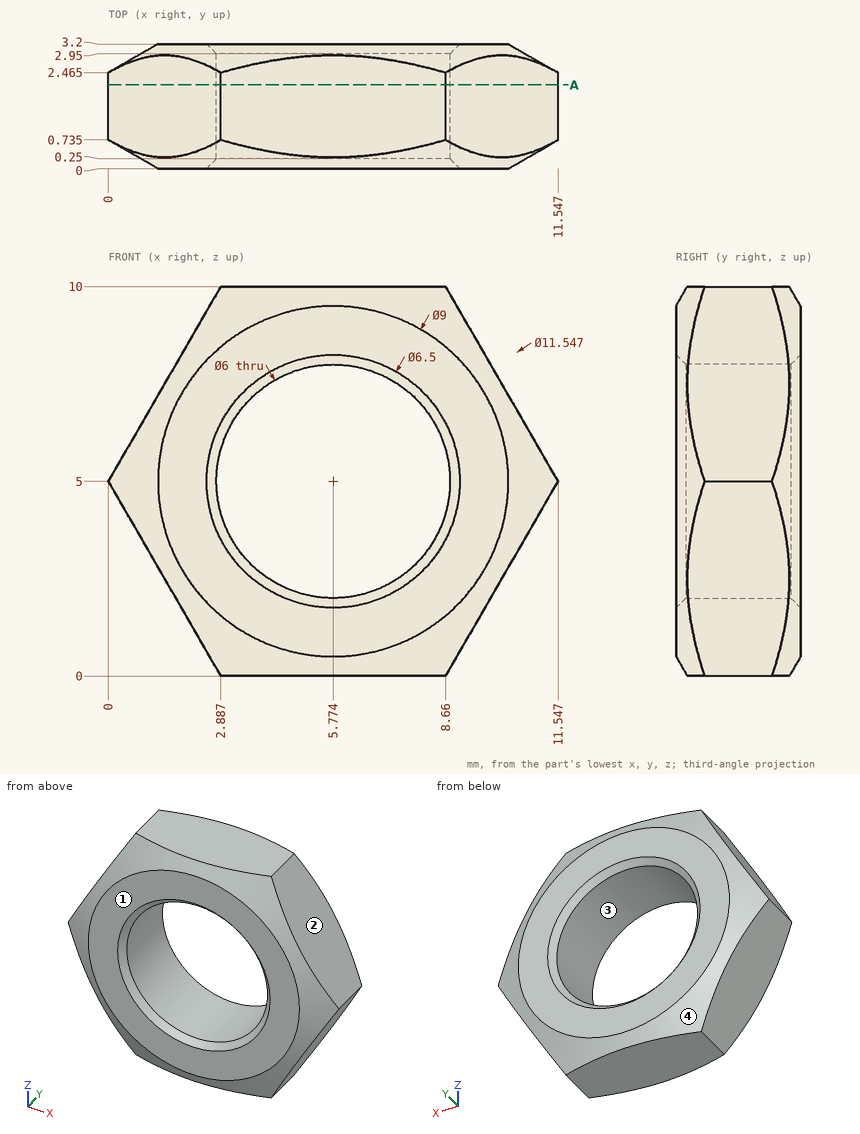
Can you work these out from the drawing? Everything is in mm from the part's minimum corner. Coordinates: 2 decimals unless noted, no trailing zeros. Loops run counter-clockwise (first coordinate to the right, second up) from the corner with the lowest first, then second, coordinate; pieces in that order, holes last. Notation, with made-up numbers: (20, 26.5) - (70, 26.5) arc R30 cw to (70, 56.5) - close; hole circle Ø11 at (-4, -9.5). An arc over 180 degrees is marked (long way). Use a Markdown table: item, result.
Item 1: If I drill on probe 1 along Z at (x, y) = (5.75, 1.1); probe 2 along Z at (x, y) = (4, 2.2); probe 3 along X at (y, z) = (1.55, 4.5) (1 decimal), over which ranges is the centre line in solid material (lowest first)? Write a range as from..to.
Numbers:
| item | result |
|---|---|
| probe 1 | z = 0..2, 8..10 |
| probe 2 | z = 0..2.58, 7.42..10 |
| probe 3 | x = 0.3..2.8, 8.7..11.3 |
Item 2: Will this pin go through, and if not, where does the flat tip stop? pin 1 (1 mm diameter, centred on x = 2, y = 2.5, fed in from -Z).
Numbers:
| item | result |
|---|---|
| pin 1 | stops at z = 0.67 |
Item 3: We'd pull the mould along Z, two halves only. Please class the marked faces 1, 2, 3 and 4: released by +Z, released by -Z, zero draft, split by the parting line, or undercut.
Numbers:
| item | result |
|---|---|
| face 1 | zero draft |
| face 2 | released by +Z |
| face 3 | undercut |
| face 4 | split by the parting line |
Item 4: I want a section at A-A on y = 2.15. Please give me the cut outline in (x, z).
Numbers:
| item | result |
|---|---|
| outline | (0, 5) - (2.89, 0) - (8.66, 0) - (11.55, 5) - (8.66, 10) - (2.89, 10) - close; hole circle Ø6 at (5.77, 5) |
